from build123d import *

# Parameters (mm, degrees)
SKETCH_1_W                     = 70
SKETCH_1_H                     = 80
EXTRUDE_1_DEPTH                = 26
SKETCH_2_W                     = 11.5
SKETCH_2_H                     = 20
CUT_EXTRUDE_1_DEPTH            = 71
SKETCH_3_W                     = 45
SKETCH_3_H                     = 20
CUT_EXTRUDE_2_DEPTH            = 71
SKETCH_4_W                     = 11.5
SKETCH_4_H                     = 20
CUT_EXTRUDE_3_DEPTH            = 71
F_5_7_5_7_DIAMETER_HOLE1_D     = 5.7
F_5_7_5_7_DIAMETER_HOLE1_DEPTH = 6
F_5_7_5_7_DIAMETER_HOLE2_D     = 5.7
F_5_7_5_7_DIAMETER_HOLE2_DEPTH = 26
F_5_7_5_7_DIAMETER_HOLE3_D     = 5.7
F_5_7_5_7_DIAMETER_HOLE3_DEPTH = 17.5
F_5_7_5_7_DIAMETER_HOLE4_D     = 5.7
F_5_7_5_7_DIAMETER_HOLE4_DEPTH = 6
F_5_7_5_7_DIAMETER_HOLE5_D     = 5.7
F_5_7_5_7_DIAMETER_HOLE5_DEPTH = 68.5
F_5_7_5_7_DIAMETER_HOLE6_D     = 5.7
F_5_7_5_7_DIAMETER_HOLE6_DEPTH = 17.5
CHAMFER_1_SIZE                 = 0.3
CHAMFER_2_SIZE                 = 0.5


with BuildPart() as part:
    # 스케치1 → 보스-돌출1 (new body)
    with BuildSketch(Plane(origin=(0, 26, 0), x_dir=(1, 0, 0), z_dir=(0, 1, 0))):
        Rectangle(SKETCH_1_W, SKETCH_1_H)
    extrude(amount=-EXTRUDE_1_DEPTH)

    # 스케치2 → 컷-돌출1 (cut, through all)
    with BuildSketch(Plane(origin=(35, 0, 0), x_dir=(0, 0, -1), z_dir=(1, 0, 0))):
        with Locations((-34.25, 16)):
            Rectangle(SKETCH_2_W, SKETCH_2_H)
    extrude(amount=-CUT_EXTRUDE_1_DEPTH, mode=Mode.SUBTRACT)

    # 스케치3 → 컷-돌출2 (cut, through all)
    with BuildSketch(Plane(origin=(35, 0, 0), x_dir=(0, 0, -1), z_dir=(1, 0, 0))):
        with Locations((0, 16)):
            Rectangle(SKETCH_3_W, SKETCH_3_H)
    extrude(amount=-CUT_EXTRUDE_2_DEPTH, mode=Mode.SUBTRACT)

    # 스케치4 → 컷-돌출3 (cut, through all)
    with BuildSketch(Plane(origin=(35, 0, 0), x_dir=(0, 0, -1), z_dir=(1, 0, 0))):
        with Locations((34.25, 16)):
            Rectangle(SKETCH_4_W, SKETCH_4_H)
    extrude(amount=-CUT_EXTRUDE_3_DEPTH, mode=Mode.SUBTRACT)

    # Ø5.7 (5.7) Diameter Hole1
    with Locations(Plane(origin=(0, 6, 0), x_dir=(1, 0, 0), z_dir=(0, 1, 0))):
        with Locations((-29.75, 34)):
            Hole(F_5_7_5_7_DIAMETER_HOLE1_D / 2, depth=F_5_7_5_7_DIAMETER_HOLE1_DEPTH)

    # Ø5.7 (5.7) Diameter Hole2
    with Locations(Plane(origin=(0, 0, 0), x_dir=(-1, 0, 0), z_dir=(0, -1, 0))):
        with Locations((-29.75, -34), (-29.75, 34), (29.75, -34)):
            Hole(F_5_7_5_7_DIAMETER_HOLE2_D / 2, depth=F_5_7_5_7_DIAMETER_HOLE2_DEPTH)

    # Ø5.7 (5.7) Diameter Hole3
    with Locations(Plane.XY.offset(-22.5)):
        with Locations((-27, 20.1)):
            Hole(F_5_7_5_7_DIAMETER_HOLE3_D / 2, depth=F_5_7_5_7_DIAMETER_HOLE3_DEPTH)

    # Ø5.7 (5.7) Diameter Hole4
    with Locations(Plane(origin=(0, 0, -28.5), x_dir=(-1, 0, 0), z_dir=(0, 0, -1))):
        with Locations((-27, 20.1)):
            Hole(F_5_7_5_7_DIAMETER_HOLE4_D / 2, depth=F_5_7_5_7_DIAMETER_HOLE4_DEPTH)

    # Ø5.7 (5.7) Diameter Hole5
    with Locations(Plane.XY.offset(28.5)):
        with Locations((-27, 20.1)):
            Hole(F_5_7_5_7_DIAMETER_HOLE5_D / 2, depth=F_5_7_5_7_DIAMETER_HOLE5_DEPTH)

    # Ø5.7 (5.7) Diameter Hole6
    with Locations(Plane(origin=(0, 0, 22.5), x_dir=(-1, 0, 0), z_dir=(0, 0, -1))):
        with Locations((-27, 20.1)):
            Hole(F_5_7_5_7_DIAMETER_HOLE6_D / 2, depth=F_5_7_5_7_DIAMETER_HOLE6_DEPTH)

    # 모따기1
    chamfer_1_edges = [part.edges().sort_by_distance(p)[0] for p in [
        (-24.15, 20.1, 22.5),
        (-24.15, 20.1, 28.5),
        (24.15, 20.1, 28.5),
        (24.15, 20.1, 22.5),
        (-26.9, 6, -34),
        (-26.9, 0, -34),
        (-32.6, 6, 34),
        (-32.6, 0, 34),
        (26.9, 6, -34),
        (26.9, 0, -34),
        (26.9, 6, 34),
        (26.9, 0, 34),
        (-24.15, 20.1, -28.5),
        (-24.15, 20.1, -22.5),
        (24.15, 20.1, -28.5),
        (24.15, 20.1, -22.5),
    ]]
    chamfer(chamfer_1_edges, length=CHAMFER_1_SIZE)

    # 모따기2
    chamfer_2_edges = [part.edges().sort_by_distance(p)[0] for p in [
        (-35, 0, 0),
        (35, 26, 25.5),
        (0, 0, 40),
        (-35, 6, 34.25),
        (0, 6, 40),
        (-35, 16, 28.5),
        (0, 26, 28.5),
        (35, 6, 34.25),
        (35, 16, 28.5),
        (35, 26, -25.5),
        (-35, 26, 25.5),
        (0, 26, 22.5),
        (-35, 16, -22.5),
        (0, 26, -22.5),
        (-35, 6, 0),
        (-35, 16, 22.5),
        (35, 16, 22.5),
        (35, 6, 0),
        (35, 16, -22.5),
        (-35, 26, -25.5),
        (35, 0, 0),
        (0, 26, -28.5),
        (-35, 6, -34.25),
        (0, 6, -40),
        (-35, 16, -28.5),
        (35, 16, -28.5),
        (35, 6, -34.25),
        (35, 3, 40),
        (-35, 3, 40),
        (-35, 3, -40),
        (35, 3, -40),
        (0, 0, -40),
    ]]
    chamfer(chamfer_2_edges, length=CHAMFER_2_SIZE)


solid = part.part
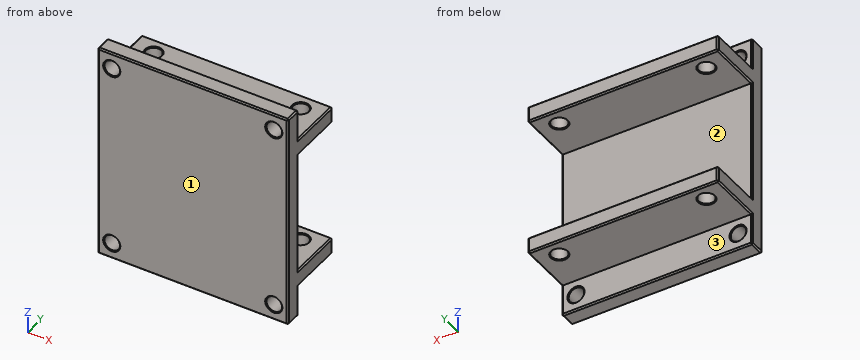
Design review of the part built by this model. Coordinates are the model's own, in mm. Face numbers are marked on the shaded views. A direction names the side the tool comes from. Round coordinates to 2 decimals unless told otherwise and drop trailing zeros. Write each loop counter-clockwise with the first axis right and the second up, starting at its lowest first coordinate (ties: lowest second). Pieces come first, ordered by that corner, then holes. Notation, with made-up numbers: (36.25, 49) - (68.25, 49) arc R9 ccw to (68.25, 55) - close; hole circle Ø2 at (34, 18). An arc over 180 degrees is marked (long way). Use a Markdown table: item, result. Add a question column.
1. Wall thickness on probe 1 along Z at (x, y) = (29.75, 4.55); probe 2 along X at (y, z) = (3.1, 34); probe 3 along Y at (x, z) = (27, -24.25): over which ranges is each line inside the solid? List them lowest first.
2. We need section C-C (x = 17). State the section outline as (y, z) points.
3. We need section D-D (z = -34). State the section outline as (x, y) points.
4. For the marked faces 1, 2 and 3, list the 3-axis set-ups (+Z, -Z, +X, -X, +Y, -Y) from which the entire face can be reached by the end or side of a thin tool; tool diameter is ignored.
5. Clearance check with flat-ended pins moving along their axes: pin 1 (4 mm diameter, centred on x = 18.5, y = 15.5, fed in from -Z); pin 2 (9 mm diameter, centred on x = -7.5, z = -36.5, fed in from +Y); pin 3 (6 mm diameter, centred on x = 0, y = 12, fed in from +Z); pin 4 (5 mm diameter, centred on x = 27, y = 20.1, fed in from -Z). State where each tip first meets the part, or that it passes through.
6. We need section A-A (y = 11.25). State the section outline as (x, z) points, then the cut area to 3 significant figures.
7. We need section B-B (y = 1.5). State the section outline as (x, z) points.
Output:
| question | item | result |
|---|---|---|
| 1 | probe 1 | z = -40 to -36.85, -31.15 to 31.15, 36.85 to 40 |
| 1 | probe 2 | x = -35 to -32.6, -26.9 to 26.9, 32.6 to 35 |
| 1 | probe 3 | y = 0 to 17.25, 22.95 to 26 |
| 2 | outline | (0, -39.5) - (0.5, -40) - (5.5, -40) - (6, -39.5) - (6, -28.5) - (25.5, -28.5) - (26, -28) - (26, -23) - (25.5, -22.5) - (6, -22.5) - (6, 22.5) - (25.5, 22.5) - (26, 23) - (26, 28) - (25.5, 28.5) - (6, 28.5) - (6, 39.5) - (5.5, 40) - (0.5, 40) - (0, 39.5) - close |
| 3 | outline | (-35, 0.5) - (-34.5, 0) - (-32.9, 0) - (-32.6, 0.3) - (-32.6, 5.7) - (-32.9, 6) - (-34.5, 6) - (-35, 5.5) - close; (-26.9, 0.3) - (-26.6, 0) - (26.6, 0) - (26.9, 0.3) - (26.9, 5.7) - (26.6, 6) - (-26.6, 6) - (-26.9, 5.7) - close; (32.6, 0.3) - (32.9, 0) - (34.5, 0) - (35, 0.5) - (35, 5.5) - (34.5, 6) - (32.9, 6) - (32.6, 5.7) - close |
| 4 | face 1 | +Z, -Z, +X, -X, -Y |
| 4 | face 2 | +X, -X, +Y |
| 4 | face 3 | -Z, +X, -X, +Y |
| 5 | pin 1 | stops at z = -28.5 |
| 5 | pin 2 | stops at y = 6 |
| 5 | pin 3 | stops at z = 28.5 |
| 5 | pin 4 | passes through |
| 6 | outline | (-35, -28) - (-34.5, -28.5) - (34.5, -28.5) - (35, -28) - (35, -23) - (34.5, -22.5) - (-34.5, -22.5) - (-35, -23) - close; (-35, 23) - (-34.5, 22.5) - (34.5, 22.5) - (35, 23) - (35, 28) - (34.5, 28.5) - (-34.5, 28.5) - (-35, 28) - close |
| 6 | area | 839 mm2 |
| 7 | outline | (-35, -39.5) - (-34.5, -40) - (34.5, -40) - (35, -39.5) - (35, 39.5) - (34.5, 40) - (-34.5, 40) - (-35, 39.5) - close; hole circle Ø5.7 at (-29.75, -34); hole circle Ø5.7 at (-29.75, 34); hole circle Ø5.7 at (29.75, -34); hole circle Ø5.7 at (29.75, 34) |
